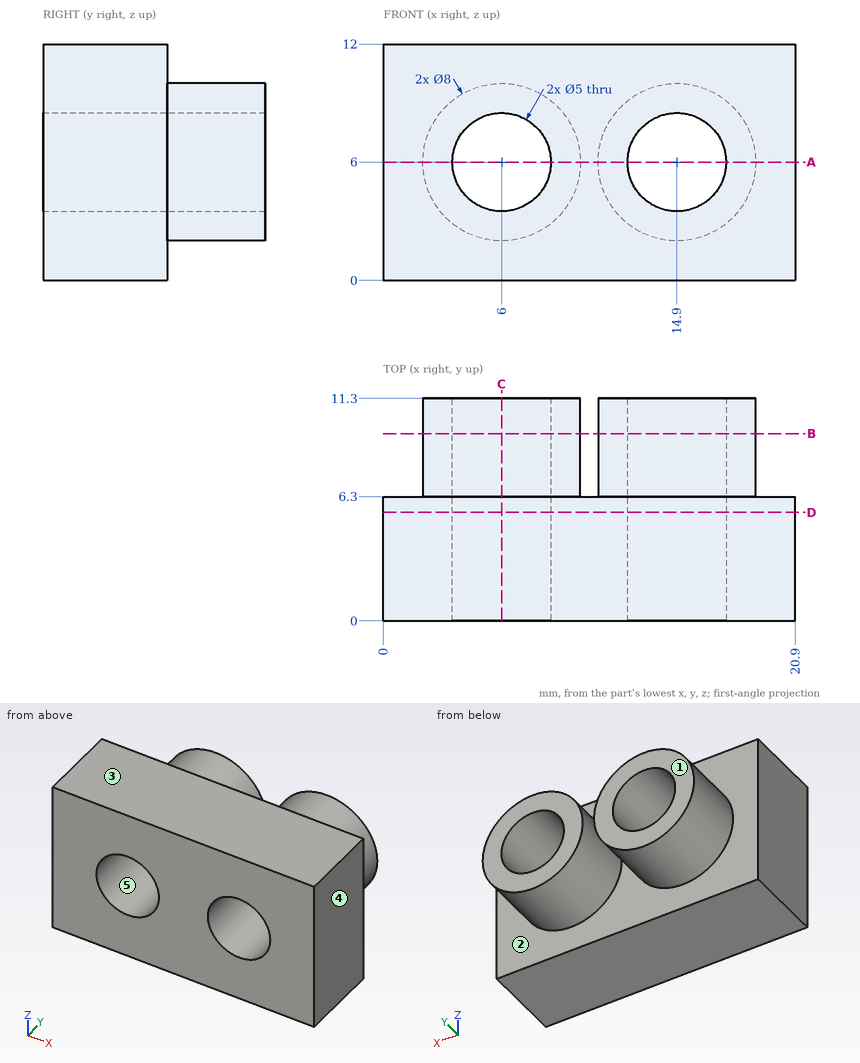
Can you work these out from the drawing? Everything is in mm from the part's minimum corner. A direction names the side the tool comes from. Round coordinates to 2 decimals unless told otherwise and drop trailing zeros. Order: outer loops, then holes, each group sorted by start corner. A loop starts at its lowest first (then second) coordinate and runs counter-clockwise, first axis right, second up.
(1) We'd pull the mould along Z, two halves only. Please class the marked faces 3, 4 and 5: +Z half, -Z half, draft (parallel to the pull), parting line (faces both ways), or undercut.
Results are:
face 3: +Z half
face 4: draft
face 5: undercut
(2) If I drill on L1, parallel to X at y = 3, z = 6; L2, parallel to X at y = 6.5, z = 6; L3, parallel to Z at x = 6, y = 8.25, over which ranges is the centre line in solid material (lowest first)?
Results are:
L1: x = 0 to 3.5, 8.5 to 12.4, 17.4 to 20.9
L2: x = 2 to 3.5, 8.5 to 10, 10.9 to 12.4, 17.4 to 18.9
L3: z = 2 to 3.5, 8.5 to 10
(3) If we section it at C-C (x = 6): Please give me the cut outline in (y, z).
Results are:
outline: (0, 0) - (6.3, 0) - (6.3, 2) - (11.3, 2) - (11.3, 3.5) - (0, 3.5) - close; (0, 8.5) - (11.3, 8.5) - (11.3, 10) - (6.3, 10) - (6.3, 12) - (0, 12) - close
(4) I'm going to push a flat-ended pin straight in: pin 1 (1 mm diameter, centred on x = 17.5, y = 9, fed in from +Z). Where does the tip first touch, or does it pass through?
Results are:
pin 1: stops at z = 9.4
(5) If we section it at D-D (y = 5.5): Please give me the cut outline in (x, z).
Results are:
outline: (0, 0) - (20.9, 0) - (20.9, 12) - (0, 12) - close; hole circle Ø5 at (6, 6); hole circle Ø5 at (14.9, 6)
(6) If we section it at A-A (z = 6): Please give me the cut outline in (x, y).
Results are:
outline: (0, 0) - (3.5, 0) - (3.5, 11.3) - (2, 11.3) - (2, 6.3) - (0, 6.3) - close; (8.5, 0) - (12.4, 0) - (12.4, 11.3) - (10.9, 11.3) - (10.9, 6.3) - (10, 6.3) - (10, 11.3) - (8.5, 11.3) - close; (17.4, 0) - (20.9, 0) - (20.9, 6.3) - (18.9, 6.3) - (18.9, 11.3) - (17.4, 11.3) - close
(7) On a 3-axis mill with a long thin cutter (end or side, diameter ignored), from which of +Z, -Z, +X, -X, +Y, -Y can I reach the whole of each face in a straight line? I mean the marked faces 1 and 2. Say none if no direction works.
Results are:
face 1: +Z, -Z, +X, -X, +Y
face 2: +Y
(8) If we section it at B-B (y = 9.5): Please give me the cut outline in (x, z), plus the area to 3 significant figures.
Results are:
outline: circle Ø8 at (6, 6); circle Ø8 at (14.9, 6); hole circle Ø5 at (6, 6); hole circle Ø5 at (14.9, 6)
area: 61.3 mm2
